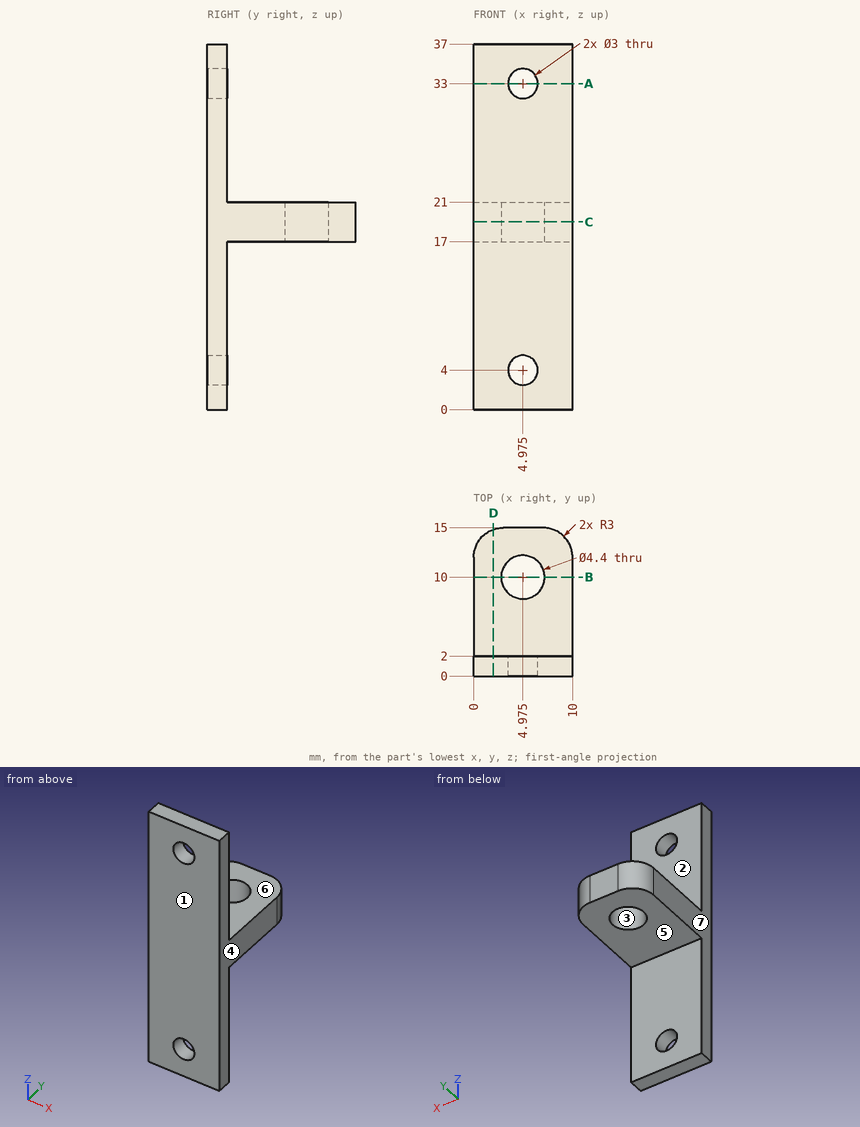
Design review of the part shown in the three views and the two pictorial views. Dimensions are in mm from the part's minimum x, y and z. A direction names the side the tool comes from. Give positions to 0.01 mm unless a question says otherwise; leave off trailing zeros. Write each loop counter-clockwise with the first axis right and the second up, starting at its lowest first coordinate (ties: lowest second). Pieces come first, ordered by that corner, then holes.
(1) Mouldability with a two-part tool opening along Y and no side actions: class the marked faces 1, 2, 3 and 4 as +Y half, -Y half, draft (parallel to the pull), parting line (faces both ways), or undercut.
Checked values:
face 1: -Y half
face 2: +Y half
face 3: undercut
face 4: draft
(2) Tool access review of the marked faces 5, 6 and 7: name each direction out of +Z, -Z, +X, -X, +Y, -Y from which nothing blocks a thin tool from reaching the whole face with its end or side.
Checked values:
face 5: -Z, +X, -X, +Y
face 6: +Z, +X, -X, +Y
face 7: +Z, -Z, -X, +Y, -Y
(3) Wall thickness on line 1 along X through (y, z) = (0.5, 33) (1 decimal); line 2 along Y through (x, z) = (3, 6); line 3 along Z through (x, y) = (1.5, 4.5): over which ranges is each line inside the solid? List them lowest first.
Checked values:
line 1: x = 0 to 3.5, 6.5 to 10
line 2: y = 0 to 2
line 3: z = 17 to 21
(4) Add section B-B (y = 10). Give the boundary of the cut face in (x, z) (1 decimal), and give its area (3 significant figures).
Checked values:
outline: (0, 17) - (2.8, 17) - (2.8, 21) - (0, 21) - close; (7.2, 17) - (10, 17) - (10, 21) - (7.2, 21) - close
area: 22.4 mm2
(5) Add section A-A (z = 33). Give the boundary of the cut face in (x, y) (1 decimal).
Checked values:
outline: (0, 0) - (3.5, 0) - (3.5, 2) - (0, 2) - close; (6.5, 0) - (10, 0) - (10, 2) - (6.5, 2) - close
(6) Clearance check with flat-ended pins moving along their axes: pin 1 Ø5.5 at (x, y) = (4.98, 10) entering from -Z; pin 2 Ø1.5 at (x, y) = (4.5, 4.5) entering from +Z; pin 3 Ø3.5 at (x, z) = (4.98, 33) entering from +Y; pin 4 Ø5 at (y, z) = (12, 25.5) entering from +X. State where each tip first meets the part, or that it passes through.
Checked values:
pin 1: stops at z = 17
pin 2: stops at z = 21
pin 3: stops at y = 2
pin 4: passes through
(7) Add section C-C (z = 19). Give the boundary of the cut face in (x, y) (1 decimal).
Checked values:
outline: (0, 0) - (10, 0) - (10, 12) arc R3 ccw to (7, 15) - (3, 15) arc R3 ccw to (0, 12) - close; hole circle Ø4.4 at (5, 10)
(8) Add section D-D (x = 2). Give the boundary of the cut face in (y, z).
Checked values:
outline: (0, 0) - (2, 0) - (2, 17) - (14.83, 17) - (14.83, 21) - (2, 21) - (2, 37) - (0, 37) - close
